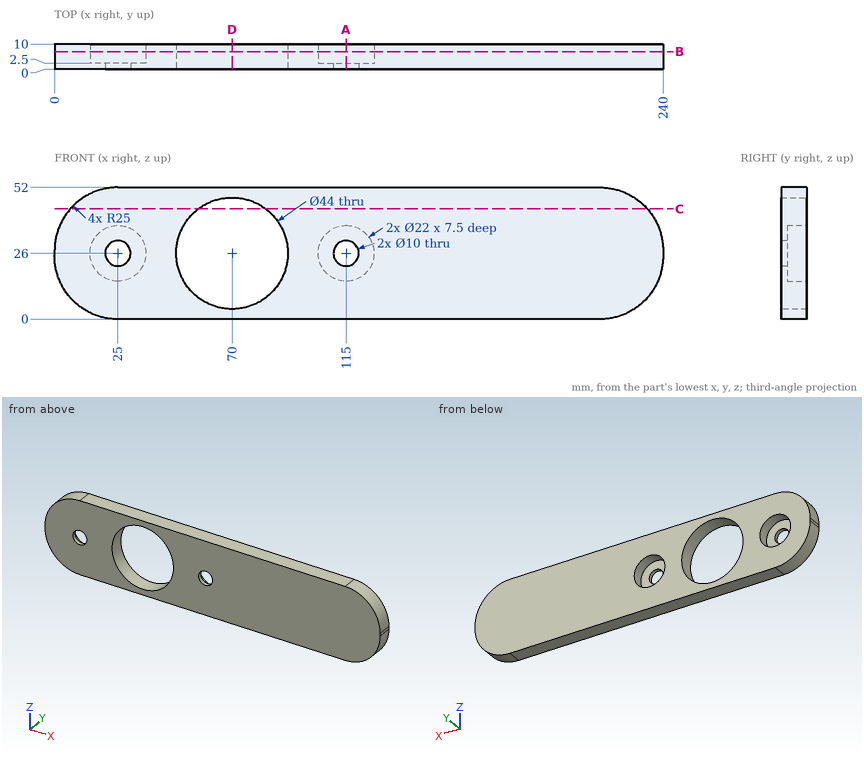
Answer from the drawing. Dimensions are ordinates in mm from the lowest x, y and z of the part. Round coordinates to 2 decimals unless told otherwise and drop trailing zeros. Order: outer loops, then holes, each group sorted by start corner. A loop starts at its lowest first (then second) coordinate and runs counter-clockwise, first axis right, second up.
1) The part is cut by section B-B on y = 7. Write down the section's boundary in (x, z), plus the area to 3 significant figures.
2) The part is cut by section D-D on x = 70. Write down the section's boundary in (y, z), plus the area to 3 significant figures.
3) Straight lines are drawn through the part: L1, parallel to X at y = 1.25, z = 26; L2, parallel to X at y = 4.5, z = 26; L3, parallel to Z at x = 25, y = 5.5. For each, find the intervals that lie inside material, in ascending order.
4) The part is cut by section C-C on z = 43.5. Write down the section's boundary in (x, y), plus the area to 3 significant figures.
5) The part is cut by section A-A on x = 115. Write down the section's boundary in (y, z), plus the area to 3 significant figures.
6) Flat-ended cylindrical pins translate along their axes: pin 1 (1.5 mm diameter, centred on y = 3.5, z = 34, fed in from -X); pin 2 (2 mm diameter, centred on y = 3.5, z = 12.5, fed in from -X); pin 3 (11 mm diameter, centred on x = 118.5, z = 24.5, fed in from +Y); pin 4 (17.5 mm diameter, centred on x = 26, z = 28.5, fed in from +Y). Find the tip coordinate at first contact, or state that the pin passes through.
Resolved:
1. outline: (0, 25) arc R25 ccw to (25, 0) - (215, 0) arc R25 ccw to (240, 25) - (240, 27) arc R25 ccw to (215, 52) - (25, 52) arc R25 ccw to (0, 27) - close; hole circle Ø22 at (25, 26); hole circle Ø44 at (70, 26); hole circle Ø22 at (115, 26)
1. area: 9,660 mm2
2. outline: (0, 0) - (10, 0) - (10, 4) - (0, 4) - close; (0, 48) - (10, 48) - (10, 52) - (0, 52) - close
2. area: 80.0 mm2
3. L1: x = 0 to 20, 30 to 48, 92 to 110, 120 to 240
3. L2: x = 0 to 14, 36 to 48, 92 to 104, 126 to 240
3. L3: z = 0 to 15, 37 to 52
4. outline: (6.22, 0) - (56.67, 0) - (56.67, 10) - (6.22, 10) - close; (83.33, 0) - (233.78, 0) - (233.78, 10) - (83.33, 10) - close
4. area: 2,010 mm2
5. outline: (0, 0) - (10, 0) - (10, 15) - (2.5, 15) - (2.5, 21) - (0, 21) - close; (0, 31) - (2.5, 31) - (2.5, 37) - (10, 37) - (10, 52) - (0, 52) - close
5. area: 330 mm2
6. pin 1: stops at x = 0.79
6. pin 2: stops at x = 2.8
6. pin 3: stops at y = 2.5
6. pin 4: stops at y = 10
